Work out the finished part from the listing and answer in its coordinate system (mm). Face numbers are marked on the shaded views. A direction names the side the tool comes from. Round coordinates to 2 decimals unless told otherwise and drop trailing zeros. Order: outer loops, then holes, each group sorted by start corner. A loop starts at its lowest first (then second) coordinate and runs counter-clockwise, first axis right, second up. Notation, with made-up numbers: (75.5, -1) -> (124.5, -1) arc R21 cw to (124.5, 19) -> close; hole circle Ø5 at (50, 10). An arc over 180 degrees is marked (long way). Use a Markdown table: item, result. Add a question column.
Item 1: Find the intervals of material crossed by L1, parallel to X at y = 5.25, z = 180; L2, parallel to Y at x = 208, z = 180; L3, parallel to X at y = 25.5, z = -174, in increasing order. Write a range as [from, to].
Item 2: A cutting plane is placed at B-B, the plane z = -109.5. Determine the outline of the cut face in (x, y).
Item 3: A tool of negligible diameter and unlimited length cuts with its end or side. For the marked faces 4 and 5, from which of +Z, -Z, +X, -X, +Y, -Y can it reach the whole face along a straight path? Write none if from no direction.
Item 4: A cutting plane is placed at D-D, the plane z = 89. Determine the outline of the cut face in (x, y), plus the area to 3 significant figures.
Item 5: A flat-ended cylindrical pin translates along its axis: P1, Ø8.5, axis at x = -120, z = 180, coming from the +Y side. Find the tip coordinate at first contact, or state that the pin passes through.
Item 6: For a pull along X with two mould halves and no side action, classify the marked faces 1, 2 and 3 as +X half, -X half, draft (parallel to the pull), parting line (faces both ways), or undercut.
Item 7: A cutting plane is placed at C-C, the plane y = 45. Determine the outline of the cut face in (x, z).
Item 8: A cutting plane is placed at A-A, the plane y = 18. Determine the outline of the cut face in (x, z), plus the area to 3 significant figures.
from build123d import *

# Parameters (mm, degrees)
EXTRUDE_THIN1_DEPTH                      = 200
CUT_EXTRUDE1_DEPTH                       = 364
SKETCH3_R                                = 5
CUT_EXTRUDE2_DEPTH                       = 417.173040934
RADYUS1_R                                = 20
M5_HELISARMAL_I_IN_Z_VANA_MATKAB_1_D     = 5.2
M5_HELISARMAL_I_IN_Z_VANA_MATKAB_1_DEPTH = 12
M5_HELISARMAL_I_IN_Z_VANA_MATKAB_1_TIP   = 1.562237609


with BuildPart() as part:
    # Sketch1 → Extrude-Thin1 (new, symmetric)
    with BuildSketch(Plane.XY):
        Polygon((-150, 60), (-150, 0), (210, 0), (210, 60), (200, 60), (200, 10), (-140, 10), (-140, 60), align=None)
    extrude(amount=EXTRUDE_THIN1_DEPTH, both=True)

    # Sketch2 → Cut-Extrude1 (cut)
    with BuildSketch(Plane(origin=(210, 0, 0), x_dir=(0, 0, -1), z_dir=(1, 0, 0))):
        with BuildLine():
            Line((40, 50), (140, 50))
            ThreePointArc((140, 50), (145, 45), (140, 40))
            Line((140, 40), (40, 40))
            ThreePointArc((40, 40), (35, 45), (40, 50))
        make_face()
    extrude(amount=-CUT_EXTRUDE1_DEPTH, mode=Mode.SUBTRACT)

    # Sketch3 → Cut-Extrude2 (cut, through all)
    with BuildSketch(Plane.ZY.offset(150)):
        with Locations((180, 45)):
            Circle(SKETCH3_R)
    extrude(amount=-CUT_EXTRUDE2_DEPTH, mode=Mode.SUBTRACT)

    # Radyus1
    radyus1_edges = [part.edges().sort_by_distance(p)[0] for p in [
        (205, 60, 200),
        (-145, 60, 200),
        (205, 60, -200),
        (-145, 60, -200),
    ]]
    fillet(radyus1_edges, radius=RADYUS1_R)

    # M5 Helisarmal için Zıvana matkabı1
    with Locations(Plane(origin=(-120, 10, 180), x_dir=(0, 0, 1), z_dir=(0, 1, 0))):
        with Locations((0, 0), (0, 300), (-360, 300), (-360, 0)):
            Hole(M5_HELISARMAL_I_IN_Z_VANA_MATKAB_1_D / 2, depth=M5_HELISARMAL_I_IN_Z_VANA_MATKAB_1_DEPTH)
            with Locations((0, 0, -(M5_HELISARMAL_I_IN_Z_VANA_MATKAB_1_DEPTH + M5_HELISARMAL_I_IN_Z_VANA_MATKAB_1_TIP / 2))):  # 118° drill point
                Cone(0, M5_HELISARMAL_I_IN_Z_VANA_MATKAB_1_D / 2, M5_HELISARMAL_I_IN_Z_VANA_MATKAB_1_TIP, mode=Mode.SUBTRACT)


solid = part.part
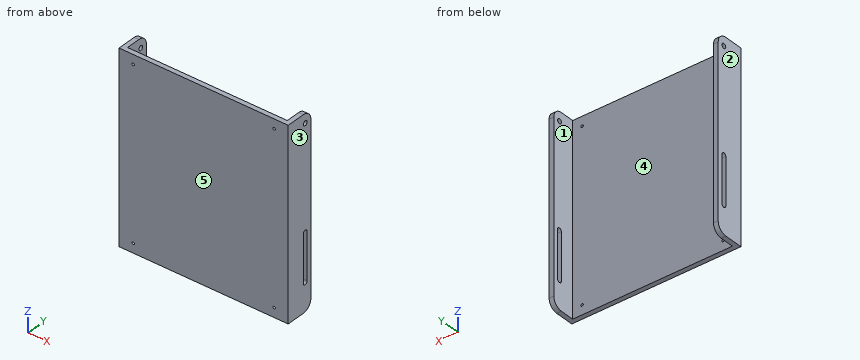
Reported:
| question | item | result |
|---|---|---|
| 1 | L1 | [-150, -122.6], [-117.4, 177.4], [182.6, 210] |
| 1 | L2 | [0, 40], [50, 60] |
| 1 | L3 | [-150, -140], [200, 210] |
| 2 | outline | (-150, 0) -> (210, 0) -> (210, 40) -> (200, 40) -> (200, 10) -> (-140, 10) -> (-140, 40) -> (-150, 40) -> close; (-150, 50) -> (-140, 50) -> (-140, 60) -> (-150, 60) -> close; (200, 50) -> (210, 50) -> (210, 60) -> (200, 60) -> close |
| 3 | face 4 | +Z, -Z, +Y |
| 3 | face 5 | +Z, -Z, +X, -X, -Y |
| 4 | outline | (-150, 0) -> (210, 0) -> (210, 60) -> (200, 60) -> (200, 10) -> (-140, 10) -> (-140, 60) -> (-150, 60) -> close |
| 4 | area | 4,600 mm² |
| 5 | P1 | y = 10 |
| 6 | face 1 | undercut |
| 6 | face 2 | -X half |
| 6 | face 3 | +X half |
| 7 | outline | (-150, -199.36) -> (-140, -199.36) -> (-140, -145) -> (-150, -145) -> close; (-150, -35) -> (-140, -35) -> (-140, 175) -> (-150, 175) -> close; (-150, 185) -> (-140, 185) -> (-140, 199.36) -> (-150, 199.36) -> close; (200, -199.36) -> (210, -199.36) -> (210, -145) -> (200, -145) -> close; (200, -35) -> (210, -35) -> (210, 175) -> (200, 175) -> close; (200, 185) -> (210, 185) -> (210, 199.36) -> (200, 199.36) -> close |
| 8 | outline | (-150, -200) -> (-140, -200) -> (-140, 200) -> (-150, 200) -> close; (200, -200) -> (210, -200) -> (210, 200) -> (200, 200) -> close |
| 8 | area | 8,000 mm² |
